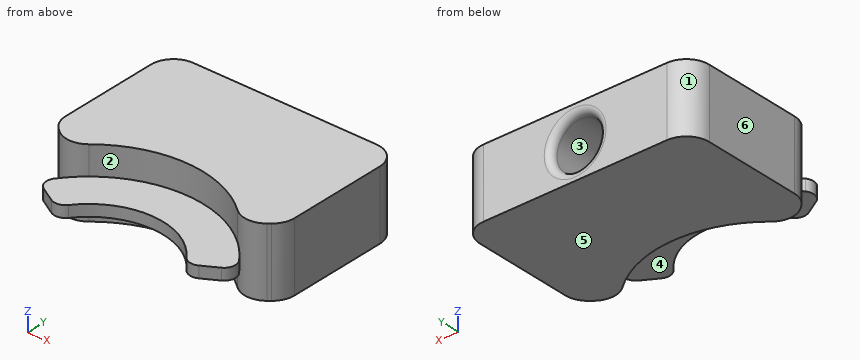
Autodesk Inventor part; units mm, degrees
ref_plane "РабПлоскость3" through (0, 0, 3) normal (0, 0, 1) x (1, 0, 0)
ref_plane "YZ Plane" through (0, 0, 0) normal (1, 0, 0) x (0, 1, 0)
ref_plane "XZ Plane" through (0, 0, 0) normal (0, 1, 0) x (-1, 0, 0)
sketch "Эскиз1" plane through (0, 0, 0) normal (0, 0, 1) x (1, 0, 0)
  line L0 (0, 0) -> (-14.5, 0)
  line L1 (14.5, 0) -> (0, 0)
  line L2 (0, -16) -> (0, 26) construction
  line L3 (-20.3, 0) -> (20.3, 0) construction
  line L4 (-10, 0) -> (-10, 20)
  line L5 (10, 0) -> (10, 20)
  line L6 (-10, 20) -> (10, 20)
  line L7 (-10, 8.391) -> (0, 0)
  line L8 (0, 0) -> (10, 8.391)
  circle A0 centre (0, 0) radius 10
  point P0 (-7.6604, 6.4279)
  point P1 (7.6604, 6.4279)
  dimension "d2" = 180
  dimension "d3" = 90
  dimension "d26" = 20
  dimension "d47" = 40
  dimension "d48" = 40
  dimension "d49" = 20
extrude "Выдавливание1" add sketch "Эскиз1" along normal blind 6 contours L7 L4 L6 L5 L8 A0
sketch "Эскиз5" plane through (-10, 20, 0) normal (0, 1, 0) x (1, 0, 0)
  line L0 (10, 0) -> (10, -6) construction
  line L1 (20, -6) -> (0, -6)
  circle A0 centre (10, -3) radius 2.1
  dimension "d50" = 4.2
extrude "Выдавливание3" cut sketch "Эскиз5" against normal blind 8
sketch "Эскиз6" plane through (0, 12, 3) normal (0, 1, 0) x (1, 0, 0)
  circle A0 centre (0, 0) radius 2.1
  circle A1 centre (0, 0) radius 1
  line L0 (0, -1) -> (0, 1)
  point P0 (0, 3)
  dimension "d53" = 2
revolve "Вращение4" cut sketch "Эскиз6" angle 360 about axis through (0, 12, 4) along (0, 0, -1) picked at (0.2078, 0.2606) contours A1 L0
fillet "Сопряжение6" radius 0.6 4 edges at (-2.1, 20, 3) (-2.1, 12, 3) (1, 12, 3) (-1, 12, 3)
fillet "Сопряжение6" radius 2 6 edges at (-7.6604, 6.4279, 3) (7.6604, 6.4279, 3) (-10, 8.391, 3) (10, 8.391, 3) (-10, 20, 3) (10, 20, 3)
ref_plane "РабПлоскость3" through (0, 0, 3) normal (0, 0, 1) x (1, 0, 0)
sketch "Эскиз7" plane through (0, 0, 3) normal (0, 0, 1) x (1, 0, 0)
  circle A0 centre (0, 0) radius 6.5
  circle A1 centre (0, 0) radius 10
  arc A2 (6.482, 7.6147) -> (-6.482, 7.6147) centre (0, 0) ccw
  line L0 (0, 0) -> (-8.6603, 5)
  line L1 (0, 0) -> (8.6603, 5)
  line L2 (-14, 0) -> (14, 0) construction
  point P0 (5.6292, 3.25)
  point P1 (-5.6292, 3.25)
  dimension "d57" = 13
  dimension "d61" = 30
  dimension "d62" = 30
extrude "Выдавливание4" add sketch "Эскиз7" along normal mid plane 1 contours A0 L0 A1 L1 picked at (4.8613, 7.3201)
fillet "Сопряжение7" radius 1 4 edges at (-5.6292, 3.25, 3) (5.6292, 3.25, 3) (8.6603, 5, 3) (-8.6603, 5, 3)
equation "\"d3\" = 0.5 * d2"
equation "\"d48\" = d47"
properties part number "Бегунок"
Build history of the part. All positions in model axes, mm. Face numbers are marked on the shaded views. A direction names the side the tool comes from. Coordinates: 2 decimals unless noted, no trailing zeros. Write each loop counter-clockwise with the first axis right and the second up, starting at its lowest first coordinate (ties: lowest second). Pieces come first, ordered by that corner, then holes.
(1) Cut at B-B on y = 5.5. List the corners of the cut face in (x, z).
(2) Pin check, flat tips, straight feed: pin 1 Ø3 at (x, z) = (1, 2) entering from -Y (3 decimals); pin 2 Ø3 at (x, y) = (3, 5.5) entering from +Z; pin 3 Ø1.9 at (x, y) = (-2.5, 7.5) entering from -Z. Stop position of each tip, or through.
(3) Cut at A-A on x = 6.75. List the corners of the cut face in (y, z).
(4) Drill centre lines: line 1 (X direction, y = 16, z = 3); line 2 (Z direction, x = 0, y = 15.5); line 3 (X direction, y = 7.5, z = 1). Where is each one in solid material? Low to high.
(5) 3-axis set-ups, long thin cutter, end or side, ignore diameter. For the marked faces 1, 2 and 3: which of +Z, -Z, +X, -X, +Y, -Y reach the whole face in a straight line?
(6) Cut at C-C on x = 8.75. List the corners of the cut face in (y, z), and give its area (3 significant figures).
(7) Mould opens along X. For the marked faces 4, 5 and 6 say: pulls with the +X half, pulls with the -X half, needs draft (parallel to the pull), parting line crosses it, or undercut.
Working result:
1. outline: (-8.23, 2.5) - (-3.46, 2.5) - (-3.46, 3.5) - (-8.23, 3.5) - close; (3.46, 2.5) - (8.23, 2.5) - (8.23, 3.5) - (3.46, 3.5) - close
2. pin 1: stops at y = 6.035
2. pin 2: stops at z = 3.5
2. pin 3: stops at z = 2.5
3. outline: (3.9, 2.5) - (7.38, 2.5) - (7.38, 3.5) - (3.9, 3.5) - close; (7.42, 0) - (20, 0) - (20, 6) - (7.42, 6) - close
4. line 1: x = -10 to -2.1, 2.1 to 10
4. line 2: z = 0 to 0.9, 5.1 to 6
4. line 3: x = -8.93 to -6.63, 6.63 to 8.93
5. face 1: +Z, -Z, -X, +Y
5. face 2: +Z, -Y
5. face 3: +Y
6. outline: (7.39, 0) - (19.85, 0) - (19.85, 6) - (7.39, 6) - close
6. area: 74.8 mm2
7. face 4: undercut
7. face 5: needs draft
7. face 6: pulls with the -X half
